Work out the finished part from the listing and answer in its coordinate system (mm). A direction names the side the tool comes from. Round coordinates to 2 decimals unless told otherwise and drop trailing zeros. Loops run counter-clockwise (first coordinate to the right, second up) from the corner with the lowest first, then second, coordinate; pieces in that order, holes last.
```python
from build123d import *

# Parameters (mm, degrees)
CUT_EXTRUDE3_DEPTH = 762
SWEEP1_START       = -76.2
SWEEP1_DEPTH       = 76.2


# Read off the part's stored shape, not the designer's step: Sweep1
with BuildPart() as part:
    # Sketch2 → Revolve3 (revolve)
    with BuildSketch(Plane.XY):
        with BuildLine():
            Line((0, 50.8), (0, -50.8))
            ThreePointArc((0, -50.8), (50.8, 0), (0, 50.8))
        make_face()
    revolve(axis=Axis((0, 50.8, 0), (0, -1, 0)))

    # Sketch2<4> → Cut-Extrude3 (cut)
    with BuildSketch(Plane.XY):
        with BuildLine():
            Line((0, 50.8), (0, -50.8))
            ThreePointArc((0, -50.8), (50.8, 0), (0, 50.8))
        make_face()
    extrude(amount=-CUT_EXTRUDE3_DEPTH, mode=Mode.SUBTRACT)

    # Sweep1 outline → Sweep1 (add)
    with BuildSketch(Plane.XY.offset(SWEEP1_START)):
        with BuildLine():
            ThreePointArc((0, -50.8), (50.8, 0), (0, 50.8))
            Line((0, 50.8), (0, -50.8))
        make_face()
    extrude(amount=SWEEP1_DEPTH)


solid = part.part
```
1. Which of the six approach directions +Z, -Z, +X, -X, +Y, -Y give full straight-line access (tool end or side, diameter ignored) to faces 1 (the face through (0, 1, -56)), 2 (the face through (50.788, -1.117, -38.633))?
Answer key:
face 1: -Z, -X
face 2: +Z, -Z, +X
2. Find section D-D (z = 19). Write down the section's boundary in (x, y), then the cut area to 3 significant figures.
Answer key:
outline: circle Ø94.23 at (0, 0)
area: 6,970 mm2
3. Consider probe 1 along Y at (x, z) = (15, -45); probe 2 along Y at (x, z) = (46, -12); probe 3 along X at (y, z) = (-1, 5). Determine where each line is inside the solid, lowest interval first.
Answer key:
probe 1: y = -48.53 to 48.53
probe 2: y = -21.56 to 21.56
probe 3: x = -50.54 to 50.54
4. Find section C-C (x = 33). Write down the section's boundary in (y, z).
Answer key:
outline: (-38.62, -76.2) - (38.62, -76.2) - (38.62, 0) arc R38.62 ccw to (-38.62, 0) - close
5. Find section B-B (y = 0). Write down the section's boundary in (x, z).
Answer key:
outline: (0, -76.2) - (50.8, -76.2) - (50.8, 0) arc R50.8 ccw (long way) to (0, -50.8) - close
6. Find section A-A (z = -53). Write down the section's boundary in (x, y), then the cut area to 3 significant figures.
Answer key:
outline: (0, -50.8) arc R50.8 ccw to (0, 50.8) - close
area: 4,050 mm2
7. Given pin 1 (8 mm diameter, centred on x = -27, z = 21, fed in from +Y); pin 2 (5 mm diameter, centred on y = -40, z = -47, fed in from -X); pin 3 (3 mm diameter, centred on x = -19, y = 35.5, fed in from +Z), each flat-ended and moving along its own axis, determine where each tip first touches the part or whether it passes through.
Answer key:
pin 1: stops at y = 40.84
pin 2: stops at x = 0
pin 3: stops at z = 32.83
